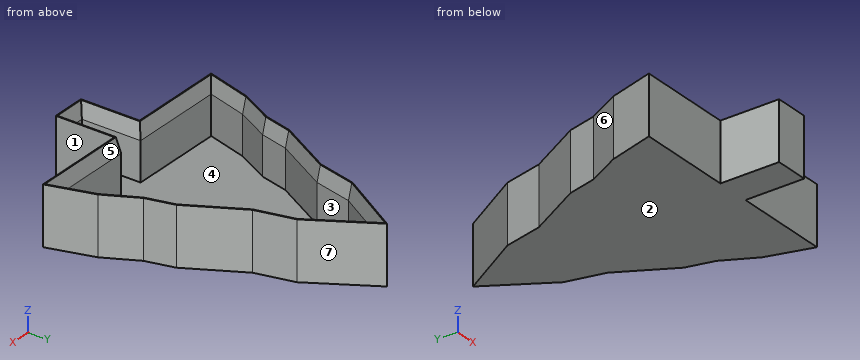
```python
from build123d import *

# Parameters (mm, degrees)
F1_DEPTH = 19.05
F2_T     = -1.27
F3_SIZE2 = 5.08
F3_SIZE  = 1.016


with BuildPart() as f1:
    # F0 (on Top) → F1 (new body)
    with BuildSketch(Plane.XY):
        Polygon((12.3290219964, 27.8594800581), (0, 48.3482889831), (-12.3290219964, 27.8594800581), (-15.2382130133, 15.3499666007), (-25.0549837339, -2.3781927895), (-27.2975303233, -11.5522462875), (-32.9452939332, -22.3343409598), (-37.2179499745, -37.2239015996), (-5.5621927604, -37.2239015996), (-5.5621927604, -56.5632171929), (0, -56.5632171929), (5.5621927604, -56.5632171929), (5.5621927604, -37.2239015996), (37.2179499745, -37.2239015996), (32.9452939332, -22.3343409598), (27.2975303233, -11.5522462875), (25.0549837339, -2.3781927895), (15.2382130133, 15.3499666007), align=None)
    extrude(amount=F1_DEPTH)

    # F2
    f2_openings = [f1.faces().sort_by_distance(p)[0] for p in [
        (0, -9.615745, 19.05),
    ]]
    offset(amount=F2_T, openings=f2_openings, kind=Kind.INTERSECTION)

    # F3
    f3_edges = [f1.edges().sort_by_distance(p)[0] for p in [
        (4.292193, -45.623559, 19.05),
        (19.912227, -35.953902, 19.05),
        (-4.292193, -45.623559, 19.05),
        (0, -55.293217, 19.05),
        (-19.912227, -35.953902, 19.05),
        (33.646255, -29.381456, 19.05),
        (28.930445, -17.406656, 19.05),
        (24.981144, -7.424546, 19.05),
        (18.951501, 6.022471, 19.05),
        (12.589404, 21.133113, 19.05),
        (5.568727, 36.630802, 19.05),
        (-5.568727, 36.630802, 19.05),
        (-12.589404, 21.133113, 19.05),
        (-18.951501, 6.022471, 19.05),
        (-24.981144, -7.424546, 19.05),
        (-28.930445, -17.406656, 19.05),
        (-33.646255, -29.381456, 19.05),
    ]]
    chamfer(f3_edges, length=F3_SIZE, length2=F3_SIZE2)


solid = f1.part
```
The model under review builds one solid part; all positions refer to its coordinate system, in mm. Face numbers are marked on the shaded views. A direction names the side the tool comes from. Round coordinates to 2 decimals unless told otherwise and drop trailing zeros. Write each loop counter-clockwise with the first axis right and the second up, starting at its lowest first coordinate (ties: lowest second). Pieces come first, ordered by that corner, then holes. Notation, with made-up numbers: (36.5, -37.75) - (71.5, -37.75) arc R28 cw to (71.5, -12.75) - close; hole circle Ø2 at (13, -12.5). An arc over 180 degrees is marked (long way). One line per question, with ' | ' between items.
Item 1: For P1, Ø9.5, axis at y = -47, z = 7.5, coming from the -X side; P2, Ø2, axis at x = 5.5, z = 7.5, coming from the +Y side; P3, Ø1, axis at y = -20.5, z = 16, coming from the -X side; P4, Ø3, axis at x = -24.5, y = -7, coming from the -Z side, all flat-tipped, find the tip position at first contact; note any pin that passes through.
Resolved:
P1: stops at x = -5.56 | P2: stops at y = 40.87 | P3: stops at x = -32.25 | P4: stops at z = 0
Item 2: The part is to be moulded in two halves that separate along X. For the marked faces 4, 5, 6 and 7, say which applies: pulls with the +X half, pulls with the -X half, needs draft (parallel to the pull), parting line crosses it, or undercut.
Resolved:
face 4: undercut | face 5: undercut | face 6: pulls with the -X half | face 7: pulls with the +X half
Item 3: To check wall thickness, follow probe 1 along X at (y, z) = (-50, 11.5); probe 2 along Z at (x, y) = (-4, -1); probe 3 along Y at (x, z) = (-9, 10.25). State the ranges of each line that lie inside material, in increasing order.
Resolved:
probe 1: x = -5.56 to -4.29, 4.29 to 5.56 | probe 2: z = 0 to 1.27 | probe 3: y = -37.22 to -35.95, 30.93 to 33.39
Item 4: Add section C-C, the plane x = 2. Give the boundary of the cut face in (y, z).
Resolved:
outline: (-56.56, 0) - (45.02, 0) - (45.02, 19.05) - (44.53, 19.05) - (42.56, 13.97) - (42.56, 1.27) - (-55.29, 1.27) - (-55.29, 13.97) - (-56.31, 19.05) - (-56.56, 19.05) - close
Item 5: Add section B-B, the plane y = -9. Give the boundary of the cut face in (x, z), then the cut area to 3 significant figures.
Resolved:
outline: (-26.67, 0) - (26.67, 0) - (26.67, 19.05) - (26.41, 19.05) - (25.37, 13.97) - (25.37, 1.27) - (-25.37, 1.27) - (-25.37, 13.97) - (-26.41, 19.05) - (-26.67, 19.05) - close | area: 109 mm2
Item 6: For the marked faces 1, 2 and 3, list the 3-axis set-ups (+Z, -Z, +X, -X, +Y, -Y) from which the entire face can be reached by the end or side of a thin tool; tool diameter is ignored.
Resolved:
face 1: +Z, -Z, +X, -Y | face 2: -Z, +X, -X, +Y, -Y | face 3: +Z
